```python
from build123d import *

# Parameters (mm, degrees)
SKETCH1_R           = 12
BOSS_EXTRUDE1_DEPTH = 8
CHAMFER1_SIZE       = 1
SKETCH2_R           = 8
BOSS_EXTRUDE2_DEPTH = 105
CHAMFER2_SIZE       = 1
SKETCH3_R           = 2
CUT_EXTRUDE1_DEPTH  = 52.5


with BuildPart() as part:
    # Sketch1 → Boss-Extrude1 (new body)
    with BuildSketch(Plane(origin=(0, 0, 0), x_dir=(0, 0, -1), z_dir=(1, 0, 0))):
        Circle(SKETCH1_R)
    extrude(amount=BOSS_EXTRUDE1_DEPTH)

    # Chamfer1
    chamfer1_edges = [part.edges().sort_by_distance(p)[0] for p in [
        (0, 0, 12),
    ]]
    chamfer(chamfer1_edges, length=CHAMFER1_SIZE)

    # Sketch2 → Boss-Extrude2 (add)
    with BuildSketch(Plane(origin=(8, 0, 0), x_dir=(0, 0, -1), z_dir=(1, 0, 0))):
        Circle(SKETCH2_R)
    extrude(amount=BOSS_EXTRUDE2_DEPTH)

    # Chamfer2
    chamfer2_edges = [part.edges().sort_by_distance(p)[0] for p in [
        (113, 0, 8),
    ]]
    chamfer(chamfer2_edges, length=CHAMFER2_SIZE)

    # Sketch3 → Cut-Extrude1 (cut, symmetric)
    with BuildSketch(Plane(origin=(0, 0, 0), x_dir=(1, 0, 0), z_dir=(0, 1, 0))):
        with Locations((102, 0)):
            Circle(SKETCH3_R)
    extrude(amount=CUT_EXTRUDE1_DEPTH, both=True, mode=Mode.SUBTRACT)


solid = part.part
```
Here's how the part is built. I have some questions about the finished solid (model axes, mm). Coordinates: 2 decimals unless noted, no trailing zeros. Order: outer loops, then holes, each group sorted by start corner. A loop starts at its lowest first (then second) coordinate and runs counter-clockwise, first axis right, second up. Notation, with made-up numbers: (65, 30.5) - (90, 30.5) arc R17 ccw to (90, 63.5) - close; hole circle Ø5 at (44, 30.5). An arc over 180 degrees is marked (long way). One line per question, with ' | ' between items.
(1) Suppose I cut it at D-D on x = 102. List the corners of the cut face in (y, z) for me, and give its area (3 significant figures).
Report:
outline: (-7.75, -2) arc R8 ccw to (7.75, -2) - close; (-7.75, 2) - (7.75, 2) arc R8 ccw to start | area: 138 mm2
(2) Will these pins go through, and if not, where does the flat tip stop? pin 1 (5 mm diameter, centred on x = 68, z = -6, fed in from -Y); pin 2 (8 mm diameter, centred on x = 62.5, z = -6, fed in from -Y); pin 3 (8 mm diameter, centred on x = 24, z = -1.5, fed in from -Y); pin 4 (3 mm diameter, centred on x = 102, z = 0, fed in from +Y).
Report:
pin 1: stops at y = -7.19 | pin 2: stops at y = -7.75 | pin 3: stops at y = -8 | pin 4: passes through
(3) Suppose I cut it at C-C on x = 85.5. List the corners of the cut face in (y, z) for me.
Report:
outline: circle Ø16 at (0, 0)
(4) Suppose I cut it at A-A on z = 0. List the corners of the cut face in (x, y) for me.
Report:
outline: (0, -11) - (1, -12) - (8, -12) - (8, -8) - (100, -8) - (100, 8) - (8, 8) - (8, 12) - (1, 12) - (0, 11) - close; (104, -8) - (112, -8) - (113, -7) - (113, 7) - (112, 8) - (104, 8) - close
(5) If we mould it in two halves opening along Z, with no side actions, what happens to faces 1 (the cylindrical face through (59.27, -7.81, 1.73)), 2 (the flat face through (8, -8, -2)), 3 (the cylindrical face through (103.908, 0.112, -0.601))? For each: pulls with the +Z half, pulls with the -Z half, needs draft (parallel to the pull), parting line crosses it, or undercut.
Report:
face 1: parting line crosses it | face 2: needs draft | face 3: undercut
(6) Suppose I cut it at B-B on y = 0. List the corners of the cut face in (x, z) for me.
Report:
outline: (0, -11) - (1, -12) - (8, -12) - (8, -8) - (112, -8) - (113, -7) - (113, 7) - (112, 8) - (8, 8) - (8, 12) - (1, 12) - (0, 11) - close; hole circle Ø4 at (102, 0)
(7) If I drill on L1, parallel to X at y = -0.5, z = 0; L2, parallel to Z at x = 102, y = 1; L3, parallel to Z at x = 102, y = 3.25, over which ranges is the centre line in solid material (lowest first)?
Report:
L1: x = 0 to 100, 104 to 113 | L2: z = -7.94 to -2, 2 to 7.94 | L3: z = -7.31 to -2, 2 to 7.31
